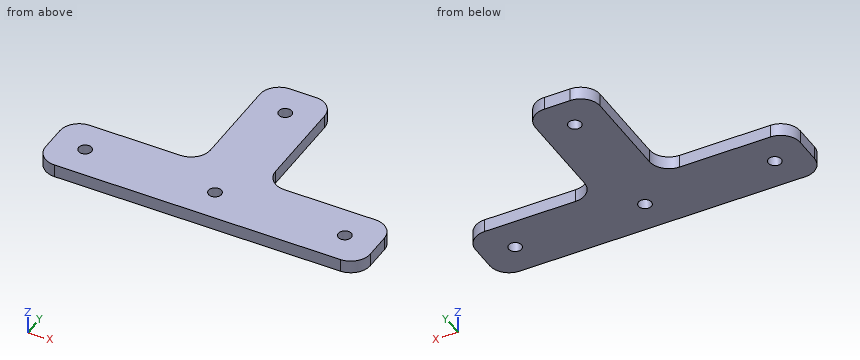
Autodesk Inventor part; units mm, degrees
ref_plane "YZ Plane" through (0, 0, 0) normal (1, 0, 0) x (0, 1, 0)
ref_plane "XZ Plane" through (0, 0, 0) normal (0, 1, 0) x (-1, 0, 0)
ref_plane "XY Plane" through (0, 0, 0) normal (0, 0, 1) x (1, 0, 0)
sketch "Szkic1" plane through (0, 0, 0) normal (0, 0, 1) x (1, 0, 0)
  line L0 (-47.736, 26.7667) -> (-47.736, 6.7667)
  line L1 (-47.736, 26.7667) -> (52.264, 26.7667)
  line L2 (52.264, 26.7667) -> (52.264, 6.7667)
  circle A0 centre (-37.736, 16.7667) radius 2
  circle A1 centre (2.264, 16.7667) radius 2
  circle A2 centre (42.264, 16.7667) radius 2
  line L3 (-7.736, 26.7667) -> (-7.736, 66.7667)
  line L4 (-7.736, 66.7667) -> (12.264, 66.7667)
  line L5 (12.264, 66.7667) -> (12.264, 26.7667)
  circle A3 centre (2.264, 56.7667) radius 2
  line L6 (-47.736, 6.7667) -> (52.264, 6.7667)
  point P0 (0, 0)
  dimension "d0" = 20
  dimension "d1" = 100
  dimension "d4" = 4
  dimension "d5" = 4
  dimension "d6" = 4
  dimension "d7" = 10
  dimension "d8" = 10
  dimension "d9" = 10
  dimension "d10" = 10
  dimension "d11" = 10
  dimension "d12" = 50
  dimension "d13" = 40
  dimension "d14" = 20
  dimension "d15" = 40
  dimension "d16" = 10
  dimension "d17" = 10
  dimension "d18" = 4
extrude "Wyciągnięcie proste1" add sketch "Szkic1" along normal blind 4
fillet "Zaokrąglenie1" radius 6 8 edges at (12.264, 26.7667, 2) (12.264, 66.7667, 2) (-7.736, 66.7667, 2) (-7.736, 26.7667, 2) (-47.736, 26.7667, 2) (52.264, 26.7667, 2) (-47.736, 6.7667, 2) (52.264, 6.7667, 2)
equation "\"d12\" = 0.5 * d1"
properties part number "LC_ALU_4mm_Heatbed_Frame_T_Bracket"
For this review, take the finished solid that the model builds, in its own axes (mm). Coordinates: 2 decimals unless noted, no trailing zeros. Loops run counter-clockwise (first coordinate to the right, second up) from the corner with the lowest first, then second, coordinate; pieces in that order, holes last.
1. Insertion check: P1, Ø1.2, axis at y = 43, z = 1.5, coming from the +X side; P2, Ø2, axis at y = 41.5, z = 3, coming from the -X side. Each pin has a flat end and moves straight along its axis. Give the tip position at first contact, or say it passes through.
2. Add section B-B, the plane x = -30. Give the boundary of the cut face in (y, z).
3. Add section C-C, the plane y = 48. Give the boundary of the cut face in (x, z).
4. For line 1 (Y direction, x = 26, z = 3.3); line 2 (X direction, y = 52, z = 0.3); line 3 (X direction, y = 29, z = 1.3), list the stretches that pass through material, from the lowest coordinate up.
5. Add section A-A, the plane z = 1.1. Give the boundary of the cut face in (x, y), then the cut area to 3 significant figures.
Result:
1. P1: stops at x = 12.26
1. P2: stops at x = -7.74
2. outline: (6.77, 0) - (26.77, 0) - (26.77, 4) - (6.77, 4) - close
3. outline: (-7.74, 0) - (12.26, 0) - (12.26, 4) - (-7.74, 4) - close
4. line 1: y = 6.77 to 26.77
4. line 2: x = -7.74 to 12.26
4. line 3: x = -9.07 to 13.59
5. outline: (-47.74, 12.77) arc R6 ccw to (-41.74, 6.77) - (46.26, 6.77) arc R6 ccw to (52.26, 12.77) - (52.26, 20.77) arc R6 ccw to (46.26, 26.77) - (18.26, 26.77) arc R6 cw to (12.26, 32.77) - (12.26, 60.77) arc R6 ccw to (6.26, 66.77) - (-1.74, 66.77) arc R6 ccw to (-7.74, 60.77) - (-7.74, 32.77) arc R6 cw to (-13.74, 26.77) - (-41.74, 26.77) arc R6 ccw to (-47.74, 20.77) - close; hole circle Ø4 at (-37.74, 16.77); hole circle Ø4 at (2.26, 16.77); hole circle Ø4 at (2.26, 56.77); hole circle Ø4 at (42.26, 16.77)
5. area: 2,720 mm2
